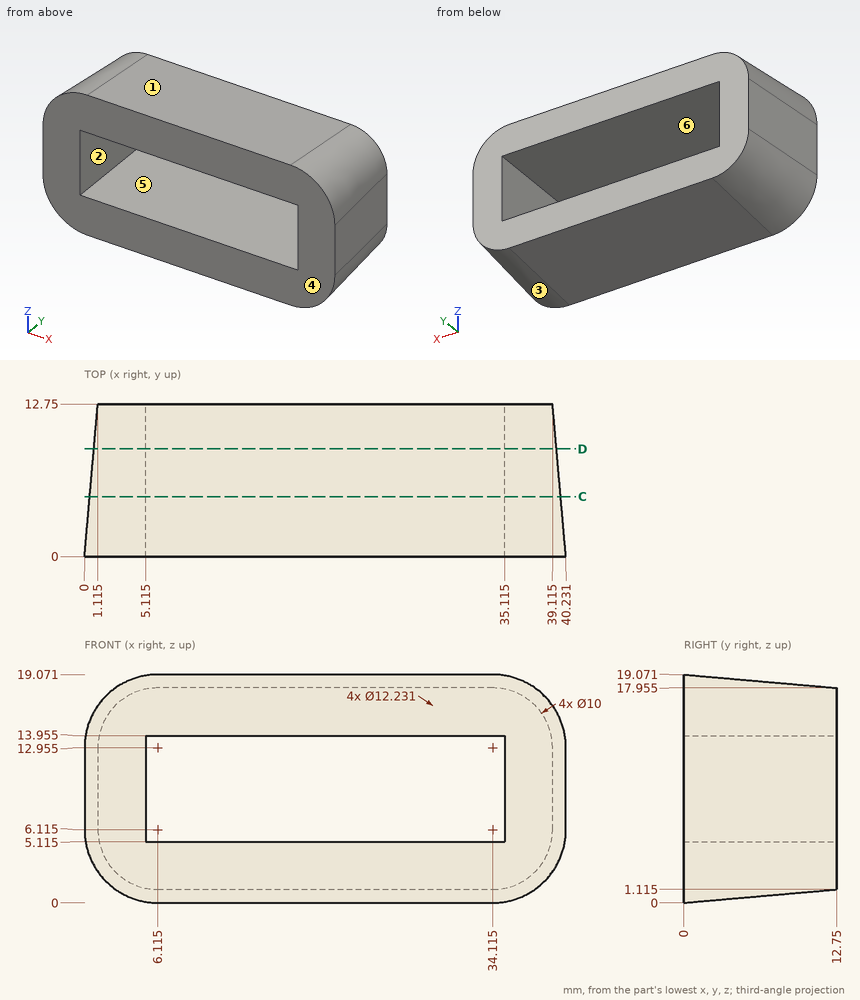
Verification items for this drawing (mm, ordinates from the low corner). A direction names the side the tool comes from. Coordinates: 2 decimals unless noted, no trailing zeros. Order: outer loops, then holes, each group sorted by start corner. A loop starts at its lowest first (then second) coordinate and runs counter-clockwise, first axis right, second up. Notation, with made-up numbers: (28, 79) - (65, 79) arc R18 ccw to (65, 92) - close; hole circle Ø3 at (87.5, 78). An arc over 180 degrees is marked (long way). Answer as a JSON object with one key per item and string values. Group by question number.
Item 1: Tool access check on the marked faces 1 and 2. Record the directions out of +Z, -Z, +X, -X, +Y, -Y that give a thin tool (end or side, any length) a straight path to the whole face; none if there is none.
Item 2: Scan lines: probe 1 along Z at (x, y) = (13.5, 4.25) (1 decimal); probe 2 along Z at (x, y) = (15, 6.5) (1 decimal); probe 3 along X at (y, z) = (11.5, 11.5) (1 decimal). Record each from-to range of solid material in increasing order.
Item 3: Draft check along X on the marked faces 3, 4, 5 and 6. Enter one of: +X half, -X half, draft (parallel to the pull), parting line (faces both ways), or undercut.
Item 4: Sectioned sample at D-D, the plane y = 9. Record the cut outline in (x, z) (1 decimal), and give its area (3 significant figures).
Item 5: Sectioned sample at C-C, the plane y = 5. Record the cut outline in (x, z) (1 decimal), and give its area (3 significant figures).
Item 6: Depth check by flat-ended pin: pin 1 Ø4 at (x, y) = (24, 6) entering from -Z; pin 2 Ø1.5 at (x, z) = (18.5, 6.5) entering from +Y; pin 3 Ø4 at (x, y) = (31, 3) entering from -Z; pin 4 Ø4 at (x, y) = (22, 6) entering from +Z. Enter the tip coordinate at first touch or a pass-through.
Resolved:
{
 "1": {"face 1": "+Z, +X, -X, +Y", "face 2": "+Y, -Y"},
 "2": {"probe 1": "0.4 to 5.1, 14 to 18.7", "probe 2": "0.6 to 5.1, 14 to 18.5", "probe 3": "1 to 5.1, 35.1 to 39.2"},
 "3": {"face 3": "+X half", "face 4": "draft", "face 5": "undercut", "face 6": "undercut"},
 "4": {"outline": "(0.8, 6.1) arc R5.3 ccw to (6.1, 0.8) - (34.1, 0.8) arc R5.3 ccw to (39.4, 6.1) - (39.4, 13) arc R5.3 ccw to (34.1, 18.3) - (6.1, 18.3) arc R5.3 ccw to (0.8, 13) - close; hole (5.1, 5.1) - (35.1, 5.1) - (35.1, 14) - (5.1, 14) - close", "area": "387 mm^2"},
 "5": {"outline": "(0.4, 6.1) arc R5.7 ccw to (6.1, 0.4) - (34.1, 0.4) arc R5.7 ccw to (39.8, 6.1) - (39.8, 13) arc R5.7 ccw to (34.1, 18.6) - (6.1, 18.6) arc R5.7 ccw to (0.4, 13) - close; hole (5.1, 5.1) - (35.1, 5.1) - (35.1, 14) - (5.1, 14) - close", "area": "423 mm^2"},
 "6": {"pin 1": "z = 0.35", "pin 2": "through", "pin 3": "z = 0.09", "pin 4": "z = 18.72"}
}
